Read the model definition and answer for the solid it produces. Units are mm, in the model's axes. Face numbers are marked on the shaded views. Give positions to 0.01 mm unless a question says otherwise; leave off trailing zeros. Write each loop counter-clockwise with the first axis right and the second up, starting at its lowest first coordinate (ties: lowest second). Pieces come first, ordered by that corner, then holes. Notation, with made-up numbers: (70, 35.5) - (98, 35.5) arc R17 cw to (98, 46.5) - close; hole circle Ø2 at (82, -20). An arc over 180 degrees is marked (long way). Answer as CSV lines item,"result".
```python
from build123d import *

# Parameters (mm, degrees)
F0_R     = 6.824609
F1_DEPTH = 12
F2_DEPTH = 31


with BuildPart() as f1:
    # F0 (on Front) → F1 (new body)
    with BuildSketch(Plane.XZ):
        with BuildLine():
            ThreePointArc((15, 50), (0, 65), (-15, 50))
            Line((-15, 50), (-15, 0))
            ThreePointArc((-15, 0), (0, 15), (15, 0))
            Line((15, 0), (15, 50))
        make_face()
        with Locations((0, 50)):
            Circle(F0_R, mode=Mode.SUBTRACT)
        with BuildLine():
            ThreePointArc((15, 0), (0, 15), (-15, 0))
            ThreePointArc((-15, 0), (0, -15), (15, 0))
        make_face()
        Circle(F0_R, mode=Mode.SUBTRACT)
    extrude(amount=-F1_DEPTH)

    # F0 (on Front) → F2 (join)
    with BuildSketch(Plane.XZ):
        with BuildLine():
            ThreePointArc((15, 0), (0, 15), (-15, 0))
            ThreePointArc((-15, 0), (0, -15), (15, 0))
        make_face()
        Circle(F0_R, mode=Mode.SUBTRACT)
    extrude(amount=-F2_DEPTH)

    # F3: F1 across face


with BuildPart() as f1_1:
    add(f1.part)
    add(f1.part.mirror(Plane(origin=(0, 31, 0), x_dir=(1, 0, 0), z_dir=(0, 1, 0))))


solid = f1_1.part
```
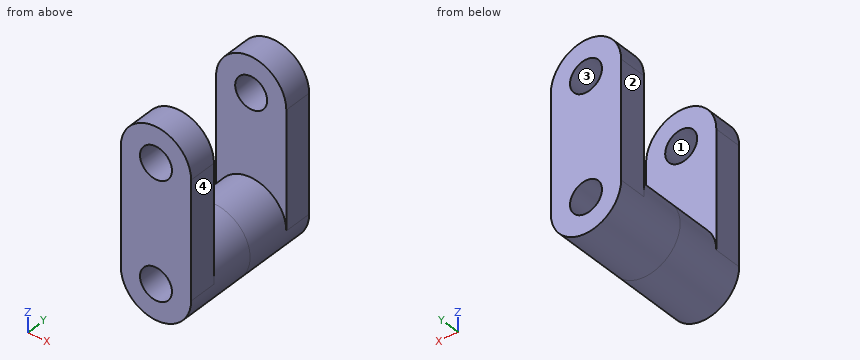
(1) A cutting plane is placed at B-B (z = 39.5). Write down the section's boundary in (x, y), and give its area (3 significant figures).
Worked out:
outline,"(-15, 0) - (15, 0) - (15, 12) - (-15, 12) - close; (-15, 50) - (15, 50) - (15, 62) - (-15, 62) - close"
area,"720 mm^2"
(2) A cutting plane is placed at A-A (x = 0). Write down the section's boundary in (y, z).
Worked out:
outline,"(0, -15) - (62, -15) - (62, -6.82) - (0, -6.82) - close; (0, 6.82) - (62, 6.82) - (62, 43.18) - (50, 43.18) - (50, 15) - (12, 15) - (12, 43.18) - (0, 43.18) - close; (0, 56.82) - (12, 56.82) - (12, 65) - (0, 65) - close; (50, 56.82) - (62, 56.82) - (62, 65) - (50, 65) - close"
(3) Each of these flat-tipped pins is pushed along its axis until it touches: P1, Ø15.5, axis at x = 0, z = 50, coming from the -Y side; P2, Ø3, axis at x = -5.5, y = 7.5, coming from the +Z side; P3, Ø3, axis at x = 3.5, y = 14.5, coming from the +Z side; P4, Ø10, axis at x = -8, y = 7, coming from the -Z side. Where does it stop, or does it pass through?
Worked out:
P1,"stops at y = 0"
P2,"stops at z = 64.46"
P3,"stops at z = 14.87"
P4,"stops at z = -14.7"
(4) Find the intervals of material crossed by L1, parallel to Z at x = 0, y = 8.25; L2, parallel to Y at x = 12, z = 11.5; L3, parallel to Z at x = 0, y = 46, in increasing order.
Worked out:
L1,"z = -15 to -6.82, 6.82 to 43.18, 56.82 to 65"
L2,"y = 0 to 12, 50 to 62"
L3,"z = -15 to -6.82, 6.82 to 15"
(5) The mould has two halves that part along X. Classify the marked faces 1, 2, 3 and 4: +X half, -X half, draft (parallel to the pull), parting line (faces both ways), or undercut.
Worked out:
face 1,"undercut"
face 2,"-X half"
face 3,"undercut"
face 4,"+X half"
(6) A cutting plane is placed at D-D (y = 36.5). Write down the section's boundary in (x, z), and give its area (3 significant figures).
Worked out:
outline,"circle Ø30 at (0, 0); hole circle Ø13.65 at (0, 0)"
area,"561 mm^2"
(7) A cutting plane is placed at C-C (y = 8). Write down the section's boundary in (x, z).
Worked out:
outline,"(-15, 0) arc R15 ccw to (15, 0) - (15, 50) arc R15 ccw to (-15, 50) - close; hole circle Ø13.65 at (0, 0); hole circle Ø13.65 at (0, 50)"
